Part model, mm, in its own coordinate system. Face numbers are marked on the shaded views. A direction names the side the tool comes from. Round coordinates to 2 decimals unless told otherwise and drop trailing zeros. Order: outer loops, then holes, each group sorted by start corner. A loop starts at its lowest first (then second) coordinate and runs counter-clockwise, first axis right, second up. Notation, with made-up numbers: (70, -6) -> (121, -6) arc R16 cw to (121, 24) -> close; hole circle Ø3 at (33.25, 12.5). An arc over 180 degrees is marked (long way). Use CSV: the item, a comma, the result in double quotes.
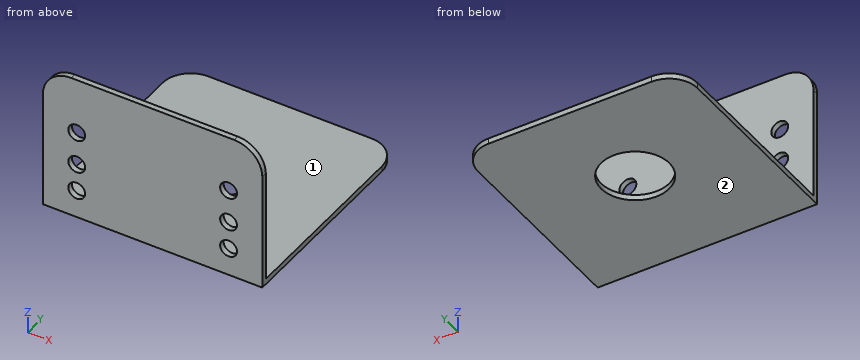
```python
from build123d import *

# Parameters (mm, degrees)
SKETCH1_W           = 39
SKETCH1_H           = 39
BOSS_EXTRUDE1_DEPTH = 1
SKETCH2_W           = 39
SKETCH2_H           = 1
BOSS_EXTRUDE2_DEPTH = 25
SKETCH5_R           = 1.5
CUT_EXTRUDE2_DEPTH  = 1
SKETCH6_R           = 1.5
CUT_EXTRUDE3_DEPTH  = 1
FILLET1_R           = 5
SKETCH7_R           = 6.05
CUT_EXTRUDE4_DEPTH  = 1


with BuildPart() as part:
    # Sketch1 → Boss-Extrude1 (new body)
    with BuildSketch(Plane.XY):
        Rectangle(SKETCH1_W, SKETCH1_H)
    extrude(amount=BOSS_EXTRUDE1_DEPTH)

    # Sketch2 → Boss-Extrude2 (add)
    with BuildSketch(Plane.XY.offset(1)):
        with Locations((0, -19)):
            Rectangle(SKETCH2_W, SKETCH2_H)
    extrude(amount=BOSS_EXTRUDE2_DEPTH)

    # Sketch5 → Cut-Extrude2 (cut)
    with BuildSketch(Plane.XZ.offset(19.5)):
        with Locations(Location((13.5, 5, 0), (0, 0, 270))):
            Circle(SKETCH5_R)
        with Locations(Location((13.5, 10, 0), (0, 0, 270))):
            Circle(SKETCH5_R)
        with Locations(Location((13.5, 16, 0), (0, 0, 270))):
            Circle(SKETCH5_R)
    extrude(amount=-CUT_EXTRUDE2_DEPTH, mode=Mode.SUBTRACT)

    # Sketch6 → Cut-Extrude3 (cut)
    with BuildSketch(Plane.XZ.offset(19.5)):
        with Locations(Location((-13.5, 16, 0), (0, 0, 270))):
            Circle(SKETCH6_R)
        with Locations(Location((-13.5, 10, 0), (0, 0, 270))):
            Circle(SKETCH6_R)
        with Locations(Location((-13.5, 5, 0), (0, 0, 270))):
            Circle(SKETCH6_R)
    extrude(amount=-CUT_EXTRUDE3_DEPTH, mode=Mode.SUBTRACT)

    # Fillet1
    fillet1_edges = [part.edges().sort_by_distance(p)[0] for p in [
        (-19.5, -19, 26),
        (19.5, -19, 26),
        (-19.5, 19.5, 0.5),
        (19.5, 19.5, 0.5),
    ]]
    fillet(fillet1_edges, radius=FILLET1_R)

    # Sketch7 → Cut-Extrude4 (cut)
    with BuildSketch(Plane.XY):
        with Locations((0, 1)):
            Circle(SKETCH7_R)
    extrude(amount=CUT_EXTRUDE4_DEPTH, mode=Mode.SUBTRACT)


solid = part.part
```
(1) Cut at A-A, the plane z = 5. Give the cut face in (x, y), then the cut area to 3 significant figures.
Reply:
outline,"(-19.5, -19.5) -> (-15, -19.5) -> (-15, -18.5) -> (-19.5, -18.5) -> close; (-12, -19.5) -> (12, -19.5) -> (12, -18.5) -> (-12, -18.5) -> close; (15, -19.5) -> (19.5, -19.5) -> (19.5, -18.5) -> (15, -18.5) -> close"
area,"33.0 mm2"
(2) Drop flat-ended pins along their axis: P1, Ø1, axis at x = -5, y = 3, coming from the -Z side; P2, Ø10, axis at x = 5, z = 10.5, coming from the +Y side; P3, Ø11.5, axis at x = -3.5, y = -4, coming from the +Z side. Give the stop position or say it passes through.
Reply:
P1,"through"
P2,"y = -18.5"
P3,"z = 1"
(3) Probe probe 1 along X at (y, z) = (-19.3, 16); probe 2 along Z at (x, y) = (-13, -19); probe 3 along Z at (x, y) = (-10, 9). List the from-to ranges inside material, lowest first. Write a range as [from, to].
Reply:
probe 1,"[-19.5, -15], [-12, 12], [15, 19.5]"
probe 2,"[0, 3.59], [6.41, 8.59], [11.41, 14.59], [17.41, 26]"
probe 3,"[0, 1]"
(4) Which spindle directions (+Z, -Z, +X, -X, +Y, -Y) get a long thin tool onto all of the face, cutting with end or side? Do the marked faces 1 and 2. Say none if no direction does.
Reply:
face 1,"+Z, +X, -X, +Y"
face 2,"-Z, +X, -X, +Y, -Y"
(5) Cut at D-D, the plane y = -17. Give the cut face in (x, z), then the cut area to 3 significant figures.
Reply:
outline,"(-19.5, 0) -> (19.5, 0) -> (19.5, 1) -> (-19.5, 1) -> close"
area,"39.0 mm2"
(6) Cut at B-B, the plane x = 0. Give the cut face in (y, z), then the cut area to 3 significant figures.
Reply:
outline,"(-19.5, 0) -> (-5.05, 0) -> (-5.05, 1) -> (-18.5, 1) -> (-18.5, 26) -> (-19.5, 26) -> close; (7.05, 0) -> (19.5, 0) -> (19.5, 1) -> (7.05, 1) -> close"
area,"51.9 mm2"
(7) Cut at C-C, the plane x = 13.5. Give the cut face in (y, z), then the cut area to 3 significant figures.
Reply:
outline,"(-19.5, 0) -> (19.5, 0) -> (19.5, 1) -> (-18.5, 1) -> (-18.5, 3.5) -> (-19.5, 3.5) -> close; (-19.5, 6.5) -> (-18.5, 6.5) -> (-18.5, 8.5) -> (-19.5, 8.5) -> close; (-19.5, 11.5) -> (-18.5, 11.5) -> (-18.5, 14.5) -> (-19.5, 14.5) -> close; (-19.5, 17.5) -> (-18.5, 17.5) -> (-18.5, 26) -> (-19.5, 26) -> close"
area,"55.0 mm2"
